from build123d import *

# Parameters (mm, degrees)
SKETCH_1_R      = 1.5
SKETCH_1_R_2    = 11.05
EXTRUDE_1_DEPTH = 1.5


with BuildPart() as part:
    # 草图1 → 凸台-拉伸1 (new body)
    with BuildSketch(Plane.XY):
        with BuildLine():
            Line((-2.598076211, 21.5), (-19.918584287, -8.5))
            ThreePointArc((-19.918584287, -8.5), (-19.918584287, -11.5), (-17.320508076, -13))
            Line((-17.320508076, -13), (17.320508076, -13))
            ThreePointArc((17.320508076, -13), (19.918584287, -11.5), (19.918584287, -8.5))
            Line((19.918584287, -8.5), (2.598076211, 21.5))
            ThreePointArc((2.598076211, 21.5), (0, 23), (-2.598076211, 21.5))
        make_face()
        with Locations((-17.320508076, -10)):
            Circle(SKETCH_1_R, mode=Mode.SUBTRACT)
        with Locations((0, 20)):
            Circle(SKETCH_1_R, mode=Mode.SUBTRACT)
        with Locations((17.320508076, -10)):
            Circle(SKETCH_1_R, mode=Mode.SUBTRACT)
        Circle(SKETCH_1_R_2, mode=Mode.SUBTRACT)
    extrude(amount=EXTRUDE_1_DEPTH)


solid = part.part
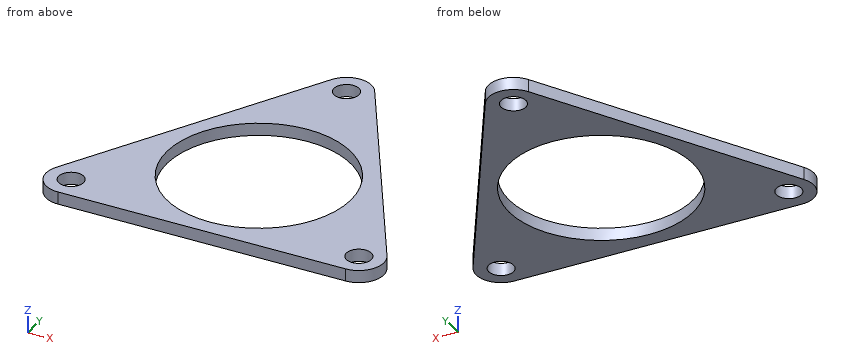
Work out the finished part from the listing and answer in its coordinate system (mm). Round coordinates to 2 decimals unless told otherwise and drop trailing zeros. Loops run counter-clockwise (first coordinate to the right, second up) from the corner with the lowest first, then second, coordinate; pieces in that order, holes last. Notation, with made-up numbers: M -30,-16 L 22,-16 A18 ccw 22,1 Z; hole C 42,-8.75 d4. An arc over 180 degrees is marked long. One line per question, with ' | ' between items. Start each with the question number.
(1) A cutting plane is placed at A-A on x = 0. Write down the section's boundary in (y, z).
(2) A cutting plane is placed at C-C on z = 1.15. Write down the section's boundary in (x, y).
(3) Find the intervals of material crossed by line 1 (Y direction, x = 0, z = 1.25); line 2 (X direction, y = 8, z = 0.95); line 3 (Y direction, x = 5.5, z = 1), in increasing order.
(4) A cutting plane is placed at B-B on y = -10. Write down the section's boundary in (x, z), plus the area to 3 significant figures.
(5) Flat-ended cylindrical pins translate along their axes: pin 1 Ø2.5 at (x, y) = (17.32, -10) entering from -Z; pin 2 Ø5 at (x, y) = (-16, 3) entering from +Z. Find the tip coordinate at first contact, or state that the pin passes through.
(6) A cutting plane is placed at D-D on y = -5. Write down the section's boundary in (x, z).
Geometry check:
1) outline: M -13,0 L -11.05,0 L -11.05,1.5 L -13,1.5 Z; M 11.05,0 L 18.5,0 L 18.5,1.5 L 11.05,1.5 Z; M 21.5,0 L 23,0 L 23,1.5 L 21.5,1.5 Z
2) outline: M -19.92,-8.5 A3 ccw -17.32,-13 L 17.32,-13 A3 ccw 19.92,-8.5 L 2.6,21.5 A3 ccw -2.6,21.5 Z; hole C -17.32,-10 d3; hole C 0,0 d22.1; hole C 0,20 d3; hole C 17.32,-10 d3
3) line 1: y = -13 to -11.05, 11.05 to 18.5, 21.5 to 23 | line 2: x = -10.39 to -7.62, 7.62 to 10.39 | line 3: y = -13 to -9.58, 9.58 to 16.47
4) outline: M -20.32,0 L -18.82,0 L -18.82,1.5 L -20.32,1.5 Z; M -15.82,0 L -4.7,0 L -4.7,1.5 L -15.82,1.5 Z; M 4.7,0 L 15.82,0 L 15.82,1.5 L 4.7,1.5 Z; M 18.82,0 L 20.32,0 L 20.32,1.5 L 18.82,1.5 Z | area: 37.9 mm²
5) pin 1: passes through | pin 2: stops at z = 1.5
6) outline: M -17.9,0 L -9.85,0 L -9.85,1.5 L -17.9,1.5 Z; M 9.85,0 L 17.9,0 L 17.9,1.5 L 9.85,1.5 Z
